from build123d import *

# Parameters (mm, degrees)
F1_DEPTH = 10


with BuildPart() as f1:
    # F0 (on Right) → F1 (new body)
    with BuildSketch(Plane.YZ):
        with BuildLine():
            Line((0, 25), (0, 0))
            Line((0, 0), (3, 0))
            Line((3, 0), (6.5, 5))
            Line((6.5, 5), (6.5, 11.535898))
            ThreePointArc((6.5, 11.535898), (4.5, 15), (6.5, 18.464102))
            Line((6.5, 18.464102), (6.5, 28.063508))
            ThreePointArc((6.5, 28.063508), (5, 30), (6.5, 31.936492))
            Line((6.5, 31.936492), (6.5, 41.763932))
            ThreePointArc((6.5, 41.763932), (5.508779, 43.770658), (6.182494, 45.905037))
            Line((6.182494, 45.905037), (1.5, 74))
            Line((1.5, 74), (0, 74))
            Line((0, 74), (0, 28))
            Line((0, 28), (2, 28))
            Line((2, 28), (2, 25))
            Line((2, 25), (0, 25))
        make_face()
    extrude(amount=F1_DEPTH)


solid = f1.part
Read the model definition and answer for the solid it produces. Units are mm, in the model's axes. A direction names the side the tool comes from. Give positions to 0.01 mm unless a question says otherwise; leave off trailing zeros. Write each loop counter-clockwise with the first axis right and the second up, starting at its lowest first coordinate (ties: lowest second). Pieces come first, ordered by that corner, then holes. Notation, with made-up numbers: (6, -3.5) -> (51, -3.5) arc R15 ccw to (51, 18.5) -> close; hole circle Ø11 at (61, 36). An arc over 180 degrees is marked (long way). Answer as a JSON object with one key per item and string values. Group by question number.
1) Find section C-C (y = 3.75). Write down the section's boundary in (x, z).
2) The mould has two halves that part along Z. Classify faces 1 (the cylindrical face through (4.93, 5.51, 43.74)), 2 (the flat face through (5, 0, 51)), 3 (the flat face through (4.93, 4.726, 2.465)), 4 (the cylindrical face through (5, 5, 30)): +Z half, -Z half, draft (parallel to the pull), parting line (faces both ways), or undercut.
3) This flat-tipped pin is pushed along its axis until it touches: P1, Ø1.5, axis at x = 6, z = 26.5, coming from the -Y side. Where does it stop, or does it pass through?
4) Consider L1, parallel to Z at x = 9.25, y = 0.5; L2, parallel to Y at x = 4, z = 58.5; L3, parallel to Y at x = 1.5, z = 52.5. Determine where each line is inside the solid, lowest interval first. Write a range as from..to.
5) Find section A-A (x = 1.5). Write down the section's boundary in (y, z).
6) A tool of negligible diameter and unlimited length cuts with its end or side. For faces 5 (the flat face through (5, 2, 27)), 6 (the flat face through (0, 2, 29)), from which of +Z, -Z, +X, -X, +Y, -Y can it reach the whole face along a straight path? Write none if from no direction.
7) Find section B-B (z = 26). Write down the section's boundary in (x, y).
Values follow:
{
 "1": {"outline": "(0, 1.07) -> (10, 1.07) -> (10, 60.5) -> (0, 60.5) -> close"},
 "2": {"face 1": "undercut", "face 2": "draft", "face 3": "-Z half", "face 4": "undercut"},
 "3": {"P1": "stops at y = 2"},
 "4": {"L1": "z = 0..25, 28..74", "L2": "y = 0..4.08", "L3": "y = 0..5.08"},
 "5": {"outline": "(0, 0) -> (3, 0) -> (6.5, 5) -> (6.5, 11.54) arc R4 cw to (6.5, 18.46) -> (6.5, 28.06) arc R2 cw to (6.5, 31.94) -> (6.5, 41.76) arc R3 cw to (6.18, 45.91) -> (1.5, 74) -> (0, 74) -> (0, 28) -> (2, 28) -> (2, 25) -> (0, 25) -> close"},
 "6": {"face 5": "+X, -X, -Y", "face 6": "+Z, -Z, -X, +Y, -Y"},
 "7": {"outline": "(0, 2) -> (10, 2) -> (10, 6.5) -> (0, 6.5) -> close"}
}
